Can you work these out from the model? Positions are in its coordinate system, mm. A direction names the side the tool comes from. Round coordinates to 2 decimals unless told otherwise and drop trailing zeros. Order: outer loops, then holes, each group sorted by start corner. A loop starts at its lowest first (then second) coordinate and runs counter-clockwise, first axis right, second up. Notation, with made-up numbers: (29, 81.5) -> (85, 81.5) arc R13 cw to (85, 86.5) -> close; hole circle Ø6 at (-6.5, 6.25). An arc over 180 degrees is marked (long way). One line per item, written item: value.
```python
from build123d import *

# Parameters (mm, degrees)
SKETCH1_R               = 15
BOSS_EXTRUDE1_DEPTH     = 10
SKETCH2_R               = 10
BOSS_EXTRUDE2_DEPTH     = 74
CUT_EXTRUDE1_DEPTH      = 74
CUT_EXTRUDE1_DEPTH_BACK = 74
SKETCH3_R               = 2.5
FILLET1_R               = 1
FILLET2_R               = 1


with BuildPart() as part:
    # Sketch1 → Boss-Extrude1 (new body)
    with BuildSketch(Plane.XY):
        Circle(SKETCH1_R)
    extrude(amount=BOSS_EXTRUDE1_DEPTH)

    # Sketch2 → Boss-Extrude2 (add)
    with BuildSketch(Plane.XY.offset(10)):
        Circle(SKETCH2_R)
    extrude(amount=BOSS_EXTRUDE2_DEPTH)

    # Sketch3 → Cut-Extrude1 (cut, two sides: drawn at the far end of the back side and taken through both)
    with BuildSketch(Plane(origin=(0, 0, 0), x_dir=(1, 0, 0), z_dir=(0, 1, 0)).offset(-CUT_EXTRUDE1_DEPTH_BACK)):
        with Locations(Location((0, -77, 0), (0, 0, 90))):
            Circle(SKETCH3_R)
    extrude(amount=CUT_EXTRUDE1_DEPTH + CUT_EXTRUDE1_DEPTH_BACK, mode=Mode.SUBTRACT)

    # Fillet1
    fillet1_edges = [part.edges().sort_by_distance(p)[0] for p in [
        (-15, 0, 0),
    ]]
    fillet(fillet1_edges, radius=FILLET1_R)

    # Fillet2
    fillet2_edges = [part.edges().sort_by_distance(p)[0] for p in [
        (-10, 0, 84),
    ]]
    fillet(fillet2_edges, radius=FILLET2_R)


solid = part.part
```
Q1. Will these pins go through, and if not, where does the flat tip stop? pin 1 Ø3 at (y, z) = (-10.5, 62.5) entering from -X; pin 2 Ø8 at (x, y) = (-7, 8.5) entering from -Z; pin 3 Ø6 at (x, z) = (0, 77) entering from +Y; pin 4 Ø2 at (x, z) = (-3, 12.5) entering from -Y.
Answers below:
pin 1: x = -4.36
pin 2: z = 0
pin 3: y = 10
pin 4: y = -9.8
Q2. We'd pull the mould along Z, two halves only. Please class faces 3 (the face through (3, -10, 10)), 4 (the face through (-14.985, 0.66, 5.437)), 5 (the face through (-0.1, -0.1, 79.5)): released by +Z, released by -Z, zero draft, split by the parting line, or undercut.
Answers below:
face 3: released by +Z
face 4: zero draft
face 5: undercut
Q3. I want a section at A-A on x = 0. List the corners of the cut face in (y, z) for me, plus the area to 3 significant figures.
Answers below:
outline: (-15, 1) arc R1 ccw to (-14, 0) -> (14, 0) arc R1 ccw to (15, 1) -> (15, 10) -> (10, 10) -> (10, 74.5) -> (-10, 74.5) -> (-10, 10) -> (-15, 10) -> close; (-10, 79.5) -> (10, 79.5) -> (10, 83) arc R1 ccw to (9, 84) -> (-9, 84) arc R1 ccw to (-10, 83) -> close
area: 1,680 mm^2
Q4. Please list where these lines run through material, in increasing order: line 1 along X through (y, z) = (0.25, 34.5); line 2 along X through (y, z) = (-2.75, 77); line 3 along Z through (x, y) = (7.5, 11).
Answers below:
line 1: -10 to 10
line 2: -9.61 to -2.5, 2.5 to 9.61
line 3: 0 to 10
Q5. I want a section at C-C on z = 76. List the corners of the cut face in (x, y) for me.
Answers below:
outline: (-2.29, -9.73) -> (-2.29, 9.73) arc R10 ccw to start; (2.29, -9.73) arc R10 ccw to (2.29, 9.73) -> close
Q6. I want a section at B-B on y = 0. List the corners of the cut face in (x, z) for me, plus the area to 3 significant figures.
Answers below:
outline: (-15, 1) arc R1 ccw to (-14, 0) -> (14, 0) arc R1 ccw to (15, 1) -> (15, 10) -> (10, 10) -> (10, 83) arc R1 ccw to (9, 84) -> (-9, 84) arc R1 ccw to (-10, 83) -> (-10, 10) -> (-15, 10) -> close; hole circle Ø5 at (0, 77)
area: 1,760 mm^2
Q7. I want a section at D-D on z = 67.5. List the corners of the cut face in (x, y) for me, plus the area to 3 significant figures.
Answers below:
outline: circle Ø20 at (0, 0)
area: 314 mm^2
Q8. On a 3-axis mill with a long thin cutter (end or side, diameter ignored), from which of +Z, -Z, +X, -X, +Y, -Y can I reach the whole of each face in a straight line? I mean faces 1 (the face through (-2.17, -9.76, 45.99)), 2 (the face through (0, 0, 84)). Say none if no direction works.
Answers below:
face 1: +Z
face 2: +Z, +X, -X, +Y, -Y
